Part model, mm, in its own coordinate system. A direction names the side the tool comes from. Give positions to 0.01 mm unless a question says otherwise; leave off trailing zeros. Order: outer loops, then holes, each group sorted by start corner. A loop starts at its lowest first (then second) coordinate and runs counter-clockwise, first axis right, second up. Notation, with made-up numbers: M 0,26.25 L 7,26.25 A10 ccw 7,36.25 Z; hole C 39.25,3.5 d9. An arc over 180 degrees is marked long. Return JSON: item names as keys, results as strings.
from build123d import *

# Parameters (mm, degrees)
SKETCH_1_R      = 22
SKETCH_1_R_2    = 3.1
SKETCH_1_R_3    = 2
EXTRUDE_1_DEPTH = 2
SKETCH_3_R      = 11
SKETCH_3_R_2    = 7.6
EXTRUDE_2_DEPTH = 7


with BuildPart() as part:
    # 草图1 → 凸台-拉伸1 (new body)
    with BuildSketch(Plane.XY):
        Circle(SKETCH_1_R)
        Circle(SKETCH_1_R_2, mode=Mode.SUBTRACT)
        with Locations((0, 16)):
            Circle(SKETCH_1_R_3, mode=Mode.SUBTRACT)
        with Locations((15.216904261, 4.94427191)):
            Circle(SKETCH_1_R_3, mode=Mode.SUBTRACT)
        with Locations((9.404564037, -12.94427191)):
            Circle(SKETCH_1_R_3, mode=Mode.SUBTRACT)
        with Locations((-9.404564037, -12.94427191)):
            Circle(SKETCH_1_R_3, mode=Mode.SUBTRACT)
        with Locations((-15.216904261, 4.94427191)):
            Circle(SKETCH_1_R_3, mode=Mode.SUBTRACT)
    extrude(amount=EXTRUDE_1_DEPTH)

    # 草图3 → 凸台-拉伸2 (add)
    with BuildSketch(Plane(origin=(0, 0, 0), x_dir=(-1, 0, 0), z_dir=(0, 0, -1))):
        with Locations(Location((0, 0, 0), (0, 0, 180))):
            Circle(SKETCH_3_R)
        Circle(SKETCH_3_R_2, mode=Mode.SUBTRACT)
    extrude(amount=EXTRUDE_2_DEPTH)


solid = part.part
Q1. Probe line 1 along Y through (x, z) = (0, 1.6); line 2 along Z through (x, y) = (-19.5, -7.5); line 3 along Y through (x, z) = (0, -3.5). List the from-to ranges inside material, lowest first.
Established:
{"line 1": "y = -22 to -3.1, 3.1 to 14, 18 to 22", "line 2": "z = 0 to 2", "line 3": "y = -11 to -7.6, 7.6 to 11"}
Q2. 3-axis set-ups, long thin cutter, end or side, ignore diameter. For faces 1 (the cylindrical face through (0, 18, 1)), 2 (the flat face through (5, 10, 0)): which of +Z, -Z, +X, -X, +Y, -Y reach the whole face in a straight line?
Established:
{"face 1": "+Z, -Z", "face 2": "-Z"}
Q3. Pin check, flat tips, straight feed: pin 1 (3 mm diameter, centred on x = -2, y = -15, fed in from -Z); pin 2 (5 mm diameter, centred on y = 13, z = 1, fed in from -X); pin 3 (3 mm diameter, centred on x = -9.4, y = -12.94, fed in from -Z); pin 4 (4.5 mm diameter, centred on x = 15.22, y = 4.94, fed in from +Z). Stop position of each tip, or through.
Established:
{"pin 1": "stops at z = 0", "pin 2": "stops at x = -19.33", "pin 3": "passes through", "pin 4": "stops at z = 2"}
Q4. Band-saw the part on A-A (x = 0). Give the cut face in (y, z), then the cut area to 3 significant figures.
Established:
{"outline": "M -22,0 L -11,0 L -11,-7 L -7.6,-7 L -7.6,0 L -3.1,0 L -3.1,2 L -22,2 Z; M 3.1,0 L 7.6,0 L 7.6,-7 L 11,-7 L 11,0 L 14,0 L 14,2 L 3.1,2 Z; M 18,0 L 22,0 L 22,2 L 18,2 Z", "area": "115 mm²"}
Q5. Two-plate mould, pull along X, no slides. Class faces 3 (the cylindrical face through (-4.769, -21.477, 0.986)), 4 (the flat face through (2.3, -7.5, -7)), 5 (the cylindrical face through (-9.66, -10.96, 0.99)): +X half, -X half, draft (parallel to the pull), parting line (faces both ways), or undercut.
Established:
{"face 3": "parting line", "face 4": "draft", "face 5": "undercut"}
Q6. Band-saw the part on D-D (x = -6). Give the cut face in (y, z), then the cut area to 3 significant figures.
Established:
{"outline": "M -21.17,0 L -9.22,0 L -9.22,-7 L -4.66,-7 L -4.66,0 L 4.66,0 L 4.66,-7 L 9.22,-7 L 9.22,0 L 21.17,0 L 21.17,2 L -21.17,2 Z", "area": "148 mm²"}
Q7. Band-saw the part on C-C (z = 0.75). Give the cut face in (x, y), then the cut area to 3 significant figures.
Established:
{"outline": "C 0,0 d44; hole C -15.22,4.94 d4; hole C -9.4,-12.94 d4; hole C 0,0 d6.2; hole C 0,16 d4; hole C 9.4,-12.94 d4; hole C 15.22,4.94 d4", "area": "1,430 mm²"}
Q8. Band-saw the part on B-B (y = -2.5). Give the cut face in (x, z), then the cut area to 3 significant figures.
Established:
{"outline": "M -21.86,0 L -10.71,0 L -10.71,-7 L -7.18,-7 L -7.18,0 L -1.83,0 L -1.83,2 L -21.86,2 Z; M 1.83,0 L 7.18,0 L 7.18,-7 L 10.71,-7 L 10.71,0 L 21.86,0 L 21.86,2 L 1.83,2 Z", "area": "130 mm²"}
